Read the model definition and answer for the solid it produces. Units are mm, in the model's axes. A direction names the side the tool comes from. Coordinates: 2 decimals unless noted, no trailing zeros. Write each loop counter-clockwise with the first axis right and the second up, starting at its lowest first coordinate (ties: lowest second). Pieces come first, ordered by that corner, then holes.
Item 1: A tool of negligible diameter and unlimited length cuts with its end or side. For faces 4 (the face through (0.605, 16, -3)), 5 (the face through (-6, 3, 8.642)), 6 (the face through (66.286, 7, -4)), 7 (the face through (68, 4, -10.392)), 8 (the face through (61.555, 3, 8)), from which of +Z, -Z, +X, -X, +Y, -Y can it reach the whole face along a straight path? Write none if from no direction.
Item 2: Each of these flat-tipped pins is pushed along its axis until it touches: P1, Ø5, axis at y = 7.5, z = 7.5, coming from the -X side; P2, Ø1.5, axis at x = 16.5, z = 11, coming from the -Y side; P3, Ø0.9, axis at y = 2, z = -15.5, coming from the +X side; P4, Ø1, axis at y = 9.5, z = -6.5, coming from the +X side. Where does it stop, or does it pass through?
Item 3: Section B-B (y = 21.5) is taken. Give the vertices of the cut face in (x, z).
Item 4: Straight lines are drawn through the part: probe 1 along X at (y, z) = (5.25, -15); probe 2 along X at (y, z) = (6.5, 3.5); probe 3 along X at (y, z) = (5.25, 1.5). For each, find the intervals that lie inside material, in ascending order.
Item 5: Section C-C (z = -15) is taken. Give the vertices of the cut face in (x, y).
Item 6: Section A-A (z = 7) is taken. Give the vertices of the cut face in (x, y).
Item 7: Section D-D (z = -5) is taken. Give the vertices of the cut face in (x, y).
Item 8: Determine the mould class of faces 1 (the face through (26, 3, -22.54)), 2 (the face through (47.005, 16, -4)), 3 (the face through (50.4, 15.9, -20.3)) for opening direction X: released by +X, released by -X, zero draft, split by the parting line, or undercut.
from build123d import *

# Parameters (mm, degrees)
SKETCH1_W           = 37.75025884
SKETCH1_H           = 38
SKETCH1_W_2         = 3
SKETCH1_H_2         = 3
SKETCH1_W_3         = 3.002099817
SKETCH1_H_3         = 3.270956242
SKETCH1_W_4         = 4.73135243
SKETCH1_H_4         = 7.795369176
BOSS_EXTRUDE1_DEPTH = 6
SKETCH2_W           = 4.72004293
SKETCH2_H           = 38
BOSS_EXTRUDE2_DEPTH = 20
FILLET1_R           = 6
SKETCH3_W           = 3.670795438
SKETCH3_H           = 13.153400434
BOSS_EXTRUDE3_DEPTH = 2
MIRROR1_OUTLINE_W   = 3.002099816
MIRROR1_OUTLINE_H   = 3.270956242
MIRROR1_OUTLINE_W_2 = 3
MIRROR1_OUTLINE_H_2 = 3
MIRROR1_DEPTH       = 6
MIRROR1_START       = 6
MIRROR1_2_DEPTH     = 20
MIRROR1_3_OUTLINE_W = 3.670795437
MIRROR1_3_OUTLINE_H = 13.153400434
MIRROR1_3_DEPTH     = 2
FILLET2_R           = 4


# Read off the part's stored shape, not the designer's step: Mirror1
with BuildPart() as part:
    # Sketch1 → Boss-Extrude1 (new body)
    # profile 1 of 3: a face of its own
    with BuildSketch(Plane(origin=(0, 0, 0), x_dir=(1, 0, 0), z_dir=(0, 1, 0))):
        with Locations((4.929687173, 3.539918032)):
            Rectangle(SKETCH1_W, SKETCH1_H)
        with Locations((-5.695183407, 15.039918032)):
            Rectangle(SKETCH1_W_2, SKETCH1_H_2, mode=Mode.SUBTRACT)
        with Locations((-5.616276245, -7.006497188)):
            Rectangle(SKETCH1_W_3, SKETCH1_H_3, mode=Mode.SUBTRACT)
    # profile 2 of 3: a face of its own
    with BuildSketch(Plane(origin=(0, 0, 0), x_dir=(1, 0, 0), z_dir=(0, 1, 0))):
        with Locations((-16.311118462, 3.815370554)):
            Rectangle(SKETCH1_W_4, SKETCH1_H_4)
    # profile 3 of 3: a face of its own
    with BuildSketch(Plane(origin=(0, 0, 0), x_dir=(1, 0, 0), z_dir=(0, 1, 0))):
        Polygon((-18.676794677, -0.082314034), (-18.676794677, 7.713055142), (-18.676794677, 10.392070771), (-22.347590115, 10.392070771), (-22.347590115, -2.761329663), (-18.676794677, -2.761329663), align=None)
    extrude(amount=BOSS_EXTRUDE1_DEPTH)

    # Sketch2 → Boss-Extrude2 (add)
    with BuildSketch(Plane(origin=(0, 6, 0), x_dir=(1, 0, 0), z_dir=(0, 1, 0))):
        with Locations((-1.755204872, 3.539918032)):
            Rectangle(SKETCH2_W, SKETCH2_H)
    extrude(amount=BOSS_EXTRUDE2_DEPTH)

    # Fillet1
    # the kernel refuses this fillet: 6 mm, written as the material it takes off along each edge
    with BuildSketch(Plane(origin=(-4.115226337, 6, -22.539918032), x_dir=(1, 0, 0), z_dir=(0, 1, 0))) as fillet1_piece_1:
        with BuildLine():
            CenterArc((FILLET1_R, -FILLET1_R), FILLET1_R, 90, 90)
            Line((0, -FILLET1_R), (0, 0))
            Line((0, 0), (FILLET1_R, 0))
        make_face()
    extrude(amount=35, mode=Mode.SUBTRACT)

    # Sketch3 → Boss-Extrude3 (add)
    with BuildSketch(Plane(origin=(0, 6, 0), x_dir=(1, 0, 0), z_dir=(0, 1, 0))):
        with Locations((-20.512192396, 3.815370554)):
            Rectangle(SKETCH3_W, SKETCH3_H)
    extrude(amount=BOSS_EXTRUDE3_DEPTH)

    # Mirror1 outline → Mirror1 (add)
    with BuildSketch(Plane(origin=(0, 0, 0), x_dir=(1, 0, 0), z_dir=(0, 1, 0))):
        Polygon((23.804816593, -15.460081968), (61.555075434, -15.460081968), (61.555075434, -0.082314034), (66.286427864, -0.082314034), (66.286427864, -2.761329663), (69.957223301, -2.761329663), (69.957223301, 10.392070771), (66.286427864, 10.392070771), (66.286427864, 7.713055142), (61.555075434, 7.713055142), (61.555075434, 22.539918032), (23.804816593, 22.539918032), align=None)
        with Locations((53.225909432, -7.006497188)):
            Rectangle(MIRROR1_OUTLINE_W, MIRROR1_OUTLINE_H, mode=Mode.SUBTRACT)
        with Locations((53.304816593, 15.039918032)):
            Rectangle(MIRROR1_OUTLINE_W_2, MIRROR1_OUTLINE_H_2, mode=Mode.SUBTRACT)
    extrude(amount=MIRROR1_DEPTH)

    # Mirror1 2 outline → Mirror1 2 (add)
    with BuildSketch(Plane(origin=(0, 0, 0), x_dir=(1, 0, 0), z_dir=(0, 1, 0)).offset(MIRROR1_START)):
        with BuildLine():
            Line((51.724859524, -15.460081968), (51.724859524, 16.539918032))
            ThreePointArc((51.724859524, 16.539918032), (50.398174323, 20.302912689), (47.004816593, 22.401804238))
            Line((47.004816593, 22.401804238), (47.004816593, -15.460081968))
            Line((47.004816593, -15.460081968), (51.724859524, -15.460081968))
        make_face()
    extrude(amount=MIRROR1_2_DEPTH)

    # Mirror1 3 outline → Mirror1 3 (add)
    with BuildSketch(Plane(origin=(0, 0, 0), x_dir=(1, 0, 0), z_dir=(0, 1, 0)).offset(MIRROR1_START)):
        with Locations((68.121825583, 3.815370554)):
            Rectangle(MIRROR1_3_OUTLINE_W, MIRROR1_3_OUTLINE_H)
    extrude(amount=MIRROR1_3_DEPTH)

    # Fillet2
    # the kernel refuses this fillet: 4 mm, written as the material it takes off along each edge
    with BuildSketch(Plane(origin=(-13.945442247, -10, 15.460081968), x_dir=(0, 0, -1), z_dir=(0, 1, 0)), Plane(origin=(-13.945442247, -10, -22.539918032), x_dir=(1, 0, 0), z_dir=(0, 1, 0))) as fillet2_piece_1:
        with BuildLine():
            CenterArc((FILLET2_R, -FILLET2_R), FILLET2_R, 90, 90)
            Line((0, -FILLET2_R), (-FILLET2_R * 0.02, -FILLET2_R))
            Line((-FILLET2_R * 0.02, -FILLET2_R), (-FILLET2_R * 0.02, FILLET2_R * 0.02))
            Line((-FILLET2_R * 0.02, FILLET2_R * 0.02), (FILLET2_R, FILLET2_R * 0.02))
            Line((FILLET2_R, FILLET2_R * 0.02), (FILLET2_R, 0))
        make_face()
    extrude(amount=26, mode=Mode.SUBTRACT)
    with BuildSketch(Plane(origin=(-22.347590115, 17.966075066, 2.761329663), x_dir=(0, 0, -1), z_dir=(0, -1, 0))) as fillet2_piece_2:
        with BuildLine():
            CenterArc((3.986430026, 4), FILLET2_R, 184.720847703, 85.279152297)
            Line((0, 3.670795437), (-0.079728601, 3.664211346))
            ThreePointArc((-0.079728601, 3.664211346), (-0.08, 1.835397719), (-0.08, 0))
            Line((-0.08, 0), (0, -0.08))
            Line((0, -0.08), (3.986430026, -0.08))
            Line((3.986430026, -0.08), (3.986430026, 0))
        make_face()
    extrude(amount=27.932150132, mode=Mode.SUBTRACT)
    with BuildSketch(Plane(origin=(-22.347590115, 8, -20.358145837), x_dir=(0, -1, 0), z_dir=(0, 0, 1))) as fillet2_piece_3:
        with BuildLine():
            CenterArc((3.986430026, 4), FILLET2_R, 184.720847703, 85.279152297)
            Line((0, 3.670795437), (-0.079728601, 3.664211346))
            ThreePointArc((-0.079728601, 3.664211346), (-0.08, 1.835397719), (-0.08, 0))
            Line((-0.08, 0), (0, -0.08))
            Line((0, -0.08), (3.986430026, -0.08))
            Line((3.986430026, -0.08), (3.986430026, 0))
        make_face()
    extrude(amount=33.085550566, mode=Mode.SUBTRACT)
    with BuildSketch(Plane(origin=(-22.347590115, -9.966075066, -10.392070771), x_dir=(1, 0, 0), z_dir=(0, 1, 0))) as fillet2_piece_4:
        with BuildLine():
            CenterArc((4, -3.986430026), FILLET2_R, 94.720847703, 85.279152297)
            Line((0, -3.986430026), (-0.08, -3.986430026))
            Line((-0.08, -3.986430026), (-0.08, 0))
            Line((-0.08, 0), (0, 0.08))
            ThreePointArc((0, 0.08), (1.835397719, 0.08), (3.664211346, 0.079728601))
            Line((3.664211346, 0.079728601), (3.670795437, 0))
        make_face()
    extrude(amount=27.932150132, mode=Mode.SUBTRACT)


solid = part.part
Established:
1. face 4: +Z, -Z, +Y
1. face 5: +Y, -Y
1. face 6: +Y
1. face 7: -Z, +X, +Y, -Y
1. face 8: +Z, +Y, -Y
2. P1: stops at x = -13.95
2. P2: stops at y = 0
2. P3: stops at x = 61.56
2. P4: stops at x = 51.72
3. outline: (-4.12, -16.54) arc R6 ccw to (0.6, -22.4) - (0.6, 15.46) - (-4.12, 15.46) - close; (47, -22.4) arc R6 ccw to (51.72, -16.54) - (51.72, 15.46) - (47, 15.46) - close
4. probe 1: x = -13.95 to -7.2, -4.2 to 51.8, 54.8 to 61.56
4. probe 2: x = -4.12 to 0.6, 47 to 51.72
4. probe 3: x = -21.28 to -18.68, -13.95 to 61.56, 66.29 to 69.96
5. outline: (-13.95, 0) - (-7.2, 0) - (-7.2, 6) - (-13.95, 6) - close; (-4.2, 0) - (51.8, 0) - (51.8, 6) - (51.72, 6) - (51.72, 26) - (47, 26) - (47, 6) - (0.6, 6) - (0.6, 26) - (-4.12, 26) - (-4.12, 6) - (-4.2, 6) - close; (54.8, 0) - (61.56, 0) - (61.56, 6) - (54.8, 6) - close
6. outline: (-13.95, 0) - (-7.12, 0) - (-7.12, 6) - (-13.95, 6) - close; (-4.12, 0) - (51.72, 0) - (51.72, 26) - (47, 26) - (47, 6) - (0.6, 6) - (0.6, 26) - (-4.12, 26) - close; (54.73, 0) - (61.56, 0) - (61.56, 6) - (54.73, 6) - close
7. outline: (-22.35, 0) - (69.96, 0) - (69.96, 8) - (66.29, 8) - (66.29, 6) - (51.72, 6) - (51.72, 26) - (47, 26) - (47, 6) - (0.6, 6) - (0.6, 26) - (-4.12, 26) - (-4.12, 6) - (-18.68, 6) - (-18.68, 8) arc R4 ccw to (-22.35, 4.01) - close
8. face 1: zero draft
8. face 2: undercut
8. face 3: released by +X
